```python
from build123d import *

# Parameters (mm, degrees)
BOSS_EXTRUDE1_DEPTH = 80
CUT_EXTRUDE2_DEPTH  = 82.280481137
SKETCH6_W           = 4
SKETCH6_H           = 13
BOSS_EXTRUDE6_DEPTH = 70
BOSS_EXTRUDE7_REACH = 148.386
BOSS_EXTRUDE8_REACH = 152.425


with BuildPart() as part:
    # Sketch1 → Boss-Extrude1 (new body)
    with BuildSketch(Plane(origin=(0, 0, 0), x_dir=(1, 0, 0), z_dir=(0, 1, 0))):
        Polygon((3.622068507, 4.197822071), (3.622068507, -8.802177929), (-0.377931493, -8.802177929), (-0.377931493, 4.197822071), (-3.677931493, 4.197822071), (-3.677931493, -8.802177929), (-7.677931493, -8.802177929), (-7.677931493, 8.878435326), align=None)
    extrude(amount=BOSS_EXTRUDE1_DEPTH)

    # Sketch2 → Cut-Extrude2 (cut, through all)
    with BuildSketch(Plane.ZY.offset(7.677931493)):
        Polygon((8.802177929, 80), (-8.878435326, 80), (-8.878435326, 72.672231838), align=None)
    extrude(amount=-CUT_EXTRUDE2_DEPTH, mode=Mode.SUBTRACT)

    # Sketch6 → Boss-Extrude6 (add, along a direction that is not the sketch's normal)
    with BuildSketch(Plane.XY.offset(8.802177929)):
        with Locations((-5.677931493, 73.5)):
            Rectangle(SKETCH6_W, SKETCH6_H)
        with Locations((1.622068507, 73.5)):
            Rectangle(SKETCH6_W, SKETCH6_H)
    extrude(amount=BOSS_EXTRUDE6_DEPTH, dir=(0, 0.38287155344466034, 0.9238015877681054))

    # Boss-Extrude7: up to this plane
    boss_extrude7_end = Plane(origin=(3.622068507, 80, -4.197822071), z_dir=(-0.3826834323650841, 0, 0.9238795325112892))
    # Sketch7 → Boss-Extrude7 (add, up to the surface)
    with BuildSketch(Plane.XY.offset(73.468289073), mode=Mode.PRIVATE) as boss_extrude7_sk1:
        Polygon((3.622068507, 106.801008741), (-7.677931493, 106.801008741), (-7.677931493, 111.481621996), align=None)
    boss_extrude7_tool1 = split(extrude(boss_extrude7_sk1.sketch, amount=BOSS_EXTRUDE7_REACH, dir=(0, -0.382871553445, -0.923801587768), mode=Mode.PRIVATE), bisect_by=boss_extrude7_end, keep=Keep.BOTH, mode=Mode.PRIVATE)
    add(boss_extrude7_tool1.solids().sort_by_distance((-3.911265, 108.361213, 73.468289))[0])

    # Boss-Extrude8: up to this plane
    boss_extrude8_end = Plane(origin=(3.622068507, 80, -4.197822071), z_dir=(-0.3826834323650841, 0, 0.9238795325112892))
    # Sketch14 → Boss-Extrude8 (add, up to the surface)
    with BuildSketch(Plane.XY.offset(73.468289073), mode=Mode.PRIVATE) as boss_extrude8_sk1:
        Polygon((7.65257716, 121.155276399), (4.824150035, 123.983703524), (-7.677931493, 111.481621996), (3.622068507, 106.801008741), (12.814456663, 115.993396897), (9.986029538, 118.821824021), (0.793641383, 109.629435866), (-1.539810995, 111.962888244), align=None)
    boss_extrude8_tool1 = split(extrude(boss_extrude8_sk1.sketch, amount=BOSS_EXTRUDE8_REACH, dir=(0, -0.382871553445, -0.923801587768), mode=Mode.PRIVATE), bisect_by=boss_extrude8_end, keep=Keep.BOTH, mode=Mode.PRIVATE)
    add(boss_extrude8_tool1.solids().sort_by_distance((6.049263, 122.380389, 73.468289))[0])

    # Mirror9: part across plane


with BuildPart() as part_1:
    add(part.part)
    add(part.part.mirror(Plane(origin=(2.014593878, 0, -4.863659863), x_dir=(0.9238795325112891, 0, 0.3826834323650842), z_dir=(0.3826834323650841, 0, -0.9238795325112892))))


solid = part_1.part
```
Source: CAD feature listing. Evaluate the final solid. Frame: model axes, mm. A direction names the side the tool comes from. Round coordinates to 2 decimals unless told otherwise and drop trailing zeros. Loops run counter-clockwise (first coordinate to the right, second up) from the corner with the lowest first, then second, coordinate; pieces in that order, holes last.
1. Access query for faces 5 (the flat face through (-0.378, 73, 18)), 6 (the flat face through (27.619, 94.354, -33.87)), 7 (the flat face through (2, 33, 8.802)), 8 (the flat face through (16.18, 72.93, -22.41)). Directions: +Z, -Z, +X, -X, +Y, -Y. A direction counts if a zero-diameter tool reaches every point of the face in a straight line with its end or side. Return the directions, or none.
2. Contact query for flat-ended pins moving along their axis: pin 1 (2 mm diameter, centred on x = 2, y = 33.5, fed in from +Z); pin 2 (3 mm diameter, centred on x = 54.5, y = 90, fed in from +Z); pin 3 (2 mm diameter, centred on x = 6, y = 62, fed in from -Z). Output: stop coordinate, or through.
3. Section query C-C on z = 28.5. Output: boundary loops of the cut face in (x, y), and give its area (3 significant figures).
4. Section query B-B on y = 30. Output: boundary loops of the cut face in (x, z).
5. Section query A-A on y = 98.5. Output: boundary loops of the cut face in (x, z), and give its area (3 significant figures).
6. Ray query, L1, parallel to X at y = 84, z = 26; L2, parallel to Y at x = 3, z = 17.5; L3, parallel to X at y = 97, z = -54. Return the intervals inside material, ascending.
7. Mould query, pull axis Y, two halves, no side actions, for faces 1 (the flat face through (11.36, 101.97, 36.13)), 2 (the flat face through (33.923, 80.213, -37.367)), 3 (the flat face through (-0.39, 94.35, 33.75)), 4 (the flat face through (-7.678, 64, 8)). Classes: released by +Y, released by -Y, zero draft, split by the parting line, or undercut.
Answers below:
1. face 5: +Z, -Y
1. face 6: none
1. face 7: +Z, +X, -X, -Y
1. face 8: -Y
2. pin 1: stops at z = 8.8
2. pin 2: stops at z = -53.72
2. pin 3: stops at z = -21.2
3. outline: (-7.68, 75.16) - (-3.68, 75.16) - (-3.68, 88.16) - (-0.38, 88.16) - (-0.38, 75.16) - (3.62, 75.16) - (3.62, 88.16) - (12.81, 97.36) - (9.99, 100.18) - (0.79, 90.99) - (-1.54, 93.33) - (7.65, 102.52) - (4.82, 105.35) - (-7.68, 92.84) - close
3. area: 261 mm2
4. outline: (-7.68, -8.88) - (4.82, -21.38) - (7.65, -18.55) - (-1.54, -9.36) - (0.79, -7.03) - (9.99, -16.22) - (12.81, -13.39) - (3.62, -4.2) - (3.62, 8.8) - (-0.38, 8.8) - (-0.38, -4.2) - (-3.68, -4.2) - (-3.68, 8.8) - (-7.68, 8.8) - close
5. outline: (-7.68, 42.15) - (4.82, 11.98) - (7.65, 18.81) - (-1.54, 40.98) - (0.79, 46.61) - (9.99, 24.44) - (12.81, 31.26) - (3.62, 53.44) - (3.62, 73.47) - (-0.38, 73.47) - (-0.38, 53.44) - (-3.68, 53.44) - (-3.68, 73.47) - (-7.68, 73.47) - close; (15.91, -14.79) - (28.4, -44.96) - (50.55, -67.11) - (53.38, -64.28) - (39.22, -50.12) - (41.55, -47.78) - (55.71, -61.94) - (58.54, -59.12) - (44.38, -44.95) - (35.19, -22.77) - (28.37, -19.94) - (37.55, -42.13) - (31.92, -39.8) - (22.74, -17.61) - close
5. area: 1,080 mm2
6. L1: x = -7.68 to -3.68, -0.38 to 3.62
6. L2: y = 70.6 to 88.64, 93.31 to 98.96
6. L3: x = 37.44 to 43.1, 47.77 to 53.42
7. face 1: released by +Y
7. face 2: released by -Y
7. face 3: undercut
7. face 4: zero draft
